Could you check a few things on this model? Use its own coordinates, in mm. Coordinates: 2 decimals unless noted, no trailing zeros. Write each loop counter-clockwise with the first axis right and the second up, starting at its lowest first coordinate (ties: lowest second). Pieces come first, ordered by that corner, then holes.
Item 1: If I drill on probe 1 along X at (y, z) = (1.6, 3.5); probe 2 along Z at (x, y) = (6.5, 0); probe 3 along Z at (x, y) = (-2, -1.6), over which ranges is the centre line in solid material (lowest first)?
Item 2: I want a section at C-C on x = -5.5. Please give me the cut outline in (y, z), then the cut area to 3 significant figures.
Item 3: I want a section at B-B on z = 14. Please give me the cut outline in (x, y), then the cut area to 3 significant figures.
Item 4: For P1, Ø1, axis at y = -2, z = 2.5, coming from the -X side; P2, Ø5, axis at x = 0, z = 17.5, coming from the +Y side, each with a flat end and sliding along its axis, tell me the tip position at first contact or that it passes through.
from build123d import *

# Parameters (mm, degrees)
F0_W     = 14.2837
F0_H     = 6
F1_DEPTH = 20
F2_SIZE2 = 19.99999
F2_SIZE  = 14.28369


# Not quite as in the source:
# - a fillet or chamfer is up to 0.001 mm smaller than in the source, because OpenCascade refuses the exact size


with BuildPart() as f1:
    # F0 (on Top) → F1 (new body)
    with BuildSketch(Plane.XY):
        Rectangle(F0_W, F0_H)
    extrude(amount=F1_DEPTH)

    # F2 (size 14.2837 and 20 in the source; OpenCascade refuses exactly that, so slightly less here)
    f2_edges = [f1.edges().sort_by_distance(p)[0] for p in [
        (-7.14185, 0, 20),
    ]]
    f2_side = f1.faces().sort_by_distance((0, 0, 20))[0]
    chamfer(f2_edges, length=F2_SIZE, length2=F2_SIZE2, reference=f2_side)


solid = f1.part
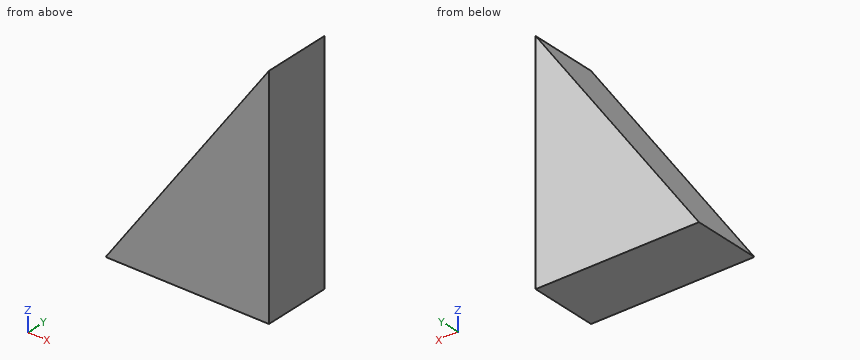
Response values:
1. probe 1: x = -4.64 to 7.14
1. probe 2: z = 0 to 19.1
1. probe 3: z = 0 to 7.2
2. outline: (-3, 0) - (3, 0) - (3, 2.3) - (-3, 2.3) - close
2. area: 13.8 mm2
3. outline: (2.86, -3) - (7.14, -3) - (7.14, 3) - (2.86, 3) - close
3. area: 25.7 mm2
4. P1: stops at x = -5.71
4. P2: passes through
